For this review, take the finished solid that the model builds, in its own axes (mm). A direction names the side the tool comes from. Round coordinates to 2 decimals unless told otherwise and drop trailing zeros. Order: outer loops, then holes, each group sorted by start corner. A loop starts at its lowest first (then second) coordinate and runs counter-clockwise, first axis right, second up. Notation, with made-up numbers: (32.5, 14.5) - (36.5, 14.5) arc R12 cw to (36.5, 34.5) - close; hole circle Ø1 at (31, -35.5). An arc over 180 degrees is marked (long way). One line per question, with ' | ' between items.
Solid Edge part; units mm, degrees
sketch "Sketch1" plane through (0, 0, 0) normal (1, 0, 0) x (0, 1, 0)
  circle A0 centre (0, 0) radius 17.5
  circle A1 centre (0, 0) radius 39.875
extrude "Protrusion1" add sketch "Sketch1" along normal mid plane 69
sketch "Sketch2" plane through (34.5, 0, 0) normal (1, 0, 0) x (0, 1, 0)
  circle A0 centre (0, 0) radius 22.5
  circle A1 centre (0, 0) radius 31
extrude "VaciadoExtruido_3" cut sketch "Sketch2" against normal blind 15
mirror "Mirror1" about plane through (0, 0, 0) normal (1, 0, 0) of "VaciadoExtruido_3"
sketch "Sketch3" plane through (34.5, 0, 0) normal (1, 0, 0) x (0, 1, 0)
  line L0 (0, 20.8) -> (-5, 20.8)
  line L1 (-5, 20.8) -> (-5, 16.7705)
  line L2 (5, 20.8) -> (5, 16.7705)
  line L3 (0, 20.8) -> (5, 20.8)
  arc A0 (-5, 16.7705) -> (5, 16.7705) centre (0, 0) cw
extrude "VaciadoExtruido_5" cut sketch "Sketch3" along normal mid plane 188
properties material "Acero"
(1) We need section A-A on z = 0. State the section outline as (x, y) points (3 decimals).
Output values:
outline: (-34.5, -39.875) - (34.5, -39.875) - (34.5, -31) - (19.5, -31) - (19.5, -22.5) - (34.5, -22.5) - (34.5, -17.5) - (-34.5, -17.5) - (-34.5, -22.5) - (-19.5, -22.5) - (-19.5, -31) - (-34.5, -31) - close; (-34.5, 17.5) - (34.5, 17.5) - (34.5, 22.5) - (19.5, 22.5) - (19.5, 31) - (34.5, 31) - (34.5, 39.875) - (-34.5, 39.875) - (-34.5, 31) - (-19.5, 31) - (-19.5, 22.5) - (-34.5, 22.5) - close
(2) Insertion check: pin 1 (4 mm diameter, centred on x = 17.5, y = -14, fed in from -Z); pin 2 (1 mm diameter, centred on x = -10.5, y = -17, fed in from -Z); pin 3 (5 mm diameter, centred on x = 11.5, y = -0.5, fed in from -Z) (3 decimals). Each pin has a flat end and moves straight along its axis. Give the tip position at first contact, or say it passes through.
Output values:
pin 1: z = -38.03 | pin 2: z = -36.3 | pin 3: z = -39.875
(3) For faces 1 (the flat face through (19.5, -9, 21)), 2 (the flat face through (34.5, -5, -17)), 3 (the flat face through (-19.5, -9, -21)), 4 (the flat face through (0, -5, 19)), 5 (the flat face through (-34.5, -5, -17)), list the 3-axis set-ups (+Z, -Z, +X, -X, +Y, -Y) from which the entire face can be reached by the end or side of a thin tool; tool diameter is ignored.
Output values:
face 1: +X | face 2: +Z, -Z, +X, +Y, -Y | face 3: -X | face 4: +X, -X | face 5: +Z, -Z, -X, +Y, -Y
(4) Mouldability with a two-part tool opening along Y and no side actions: class faces 6 (the flat face through (-34.5, 20, -24)), 7 (the cylindrical face through (27.105, 10.382, -19.961)), 8 (the cylindrical face through (-0.483, -31.643, 24.263)) as released by +Y, released by -Y, zero draft, split by the parting line, or undercut.
Output values:
face 6: zero draft | face 7: undercut | face 8: split by the parting line
(5) For probe 1 along Z at (x, y) = (27, 0) (3 decimals); probe 2 along Z at (x, y) = (-15.5, 0) (3 decimals); probe 3 along Z at (x, y) = (30, -10.5), list the stretches that pass through material, from the lowest coordinate up. Write a range as [from, to].
Output values:
probe 1: [-39.875, -31], [-22.5, -17.5], [20.8, 22.5], [31, 39.875] | probe 2: [-39.875, -17.5], [20.8, 39.875] | probe 3: [-38.47, -29.17], [-19.9, -14], [14, 19.9], [29.17, 38.47]
(6) We need section D-D on y = -27.5. State the section outline as (x, z) points (3 decimals).
Output values:
outline: (-34.5, -28.875) - (34.5, -28.875) - (34.5, -14.309) - (19.5, -14.309) - (19.5, 14.309) - (34.5, 14.309) - (34.5, 28.875) - (-34.5, 28.875) - (-34.5, 14.309) - (-19.5, 14.309) - (-19.5, -14.309) - (-34.5, -14.309) - close
(7) We need section B-B on y = 0. State the section outline as (x, z) points (3 decimals).
Output values:
outline: (-34.5, -39.875) - (34.5, -39.875) - (34.5, -31) - (19.5, -31) - (19.5, -22.5) - (34.5, -22.5) - (34.5, -17.5) - (-34.5, -17.5) - (-34.5, -22.5) - (-19.5, -22.5) - (-19.5, -31) - (-34.5, -31) - close; (-34.5, 20.8) - (34.5, 20.8) - (34.5, 22.5) - (19.5, 22.5) - (19.5, 31) - (34.5, 31) - (34.5, 39.875) - (-34.5, 39.875) - (-34.5, 31) - (-19.5, 31) - (-19.5, 22.5) - (-34.5, 22.5) - close
